```python
from build123d import *

# Parameters (mm, degrees)
SKETCH1_W                                         = 146.05
SKETCH1_H                                         = 95.25
BOSS_EXTRUDE1_DEPTH                               = 3.175
F_6_CLEARANCE_HOLE1_D                             = 4.3053
SKETCH5_R                                         = 6.35
SKETCH5_R_2                                       = 4.7625
CUT_EXTRUDE1_DEPTH                                = 8.4676
CSK_FOR_6_FLAT_HEAD_MACHINE_SCREW_100_D           = 4.3053
CSK_FOR_6_FLAT_HEAD_MACHINE_SCREW_100_CSINK_D     = 7.0866
CSK_FOR_6_FLAT_HEAD_MACHINE_SCREW_100_CSINK_ANGLE = 100
SKETCH8_R                                         = 1.134488875
CUT_EXTRUDE2_DEPTH                                = 4.175


with BuildPart() as part:
    # Sketch1 → Boss-Extrude1 (new body)
    with BuildSketch(Plane.XY):
        with Locations((-73.025, 47.625)):
            Rectangle(SKETCH1_W, SKETCH1_H)
    extrude(amount=-BOSS_EXTRUDE1_DEPTH)

    # #6 Clearance Hole1 (through all)
    with Locations(Plane(origin=(0, 0, -3.175), x_dir=(-1, 0, 0), z_dir=(0, 0, -1))):
        with Locations((4.8895, 80.9625), (141.1605, 80.9625), (141.1605, 14.2875), (4.8895, 14.2875), (46.99, 9.525), (85.725, 9.525), (97.79, 82.55), (46.99, 82.55)):
            Hole(F_6_CLEARANCE_HOLE1_D / 2)

    # Sketch5 → Cut-Extrude1 (cut, through all)
    with BuildSketch(Plane(origin=(0, 0, -7.4676), x_dir=(-1, 0, 0), z_dir=(0, 0, -1))):
        with Locations((30.988, 66.675)):
            Circle(SKETCH5_R)
        with Locations((113.03, 66.675)):
            Circle(SKETCH5_R)
        with Locations((64.5795, 20.955)):
            Circle(SKETCH5_R)
        with Locations((31.242, 20.955)):
            Circle(SKETCH5_R)
        with Locations((73.025, 68.326)):
            Circle(SKETCH5_R_2)
        with Locations((104.775, 21.59)):
            Circle(SKETCH5_R_2)
    extrude(amount=-CUT_EXTRUDE1_DEPTH, mode=Mode.SUBTRACT)

    # CSK for #6 Flat Head Machine Screw (100)1 (through all)
    with Locations(Plane(origin=(0, 0, -3.175), x_dir=(-1, 0, 0), z_dir=(0, 0, -1))):
        with Locations((90.4875, 43.815), (90.4875, 18.415), (119.0625, 7.636172046), (119.0625, 18.415), (119.0625, 43.815), (128.5875, 43.815)):
            CounterSinkHole(CSK_FOR_6_FLAT_HEAD_MACHINE_SCREW_100_D / 2, CSK_FOR_6_FLAT_HEAD_MACHINE_SCREW_100_CSINK_D / 2, counter_sink_angle=CSK_FOR_6_FLAT_HEAD_MACHINE_SCREW_100_CSINK_ANGLE)

    # Sketch8 → Cut-Extrude2 (cut, through all)
    with BuildSketch(Plane.XY):
        with Locations((-70.012401844, 73.606641948)):
            Circle(SKETCH8_R)
    extrude(amount=-CUT_EXTRUDE2_DEPTH, mode=Mode.SUBTRACT)


solid = part.part
```
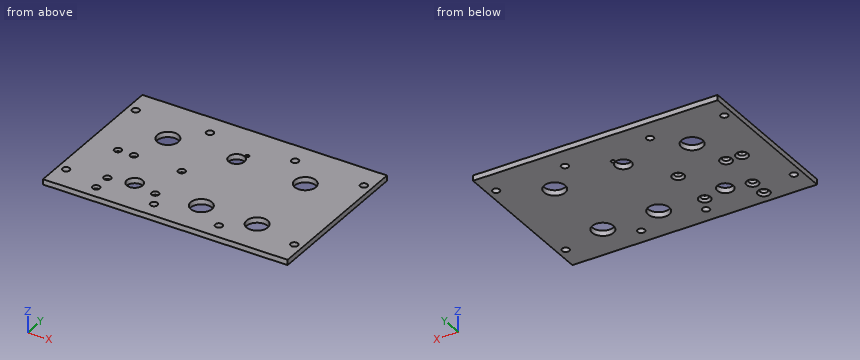
Verification items for the finished model (mm, model axes). Coordinates: 2 decimals unless noted, no trailing zeros. Order: outer loops, then holes, each group sorted by start corner. A loop starts at its lowest first (then second) coordinate and runs counter-clockwise, first axis right, second up. Notation, with made-up numbers: (-38.75, 70.25) -> (6.25, 70.25) arc R21 cw to (6.25, 87.25) -> close; hole circle Ø9 at (-26, 33). An arc over 180 degrees is marked (long way). Put each result on its own line as item: value. Start each with the question number.
1) Cross-section at B-B (y = 24). Enter the section's corners in (x, z) (3 decimals).
2) Cross-section at A-A (x = -97.79). Enter the section's corners in (y, z) (3 decimals), plus the area to 3 significant figures.
3) Material ranges on L1, parallel to X at y = 68, z = -2.05; L2, parallel to Y at x = -25.5, z = -1.7; L3, parallel to X at y = 63, z = -0.4, recorded low to high.
4) Cross-section at D-D (x = -113.03). Enter the section's corners in (y, z) (3 decimals).
5) Go/stop test with a flat-tipped pin: pin 1 (16.5 mm diameter, centred on x = -64.58, y = 20.96, fed in from +Z). Record where the tip stops, or that it passes through.
6) Cross-section at C-C (z = -2.65). State how many separate pieces and enclosed holes the cut face has, plus the area to 3 significant figures.
Geometry check:
1. outline: (-146.05, -3.175) -> (-108.883, -3.175) -> (-108.883, 0) -> (-146.05, 0) -> close; (-100.667, -3.175) -> (-70.152, -3.175) -> (-70.152, 0) -> (-100.667, 0) -> close; (-59.007, -3.175) -> (-36.814, -3.175) -> (-36.814, 0) -> (-59.007, 0) -> close; (-25.67, -3.175) -> (0, -3.175) -> (0, 0) -> (-25.67, 0) -> close
2. outline: (0, -3.175) -> (80.397, -3.175) -> (80.397, 0) -> (0, 0) -> close; (84.703, -3.175) -> (95.25, -3.175) -> (95.25, 0) -> (84.703, 0) -> close
2. area: 289 mm^2
3. L1: x = -146.05 to -119.24, -106.82 to -77.78, -68.27 to -37.2, -24.78 to 0
3. L2: y = 0 to 18.24, 23.67 to 63.48, 69.87 to 95.25
3. L3: x = -146.05 to -118.21, -107.85 to -36.17, -25.81 to 0
4. outline: (0, -3.175) -> (60.325, -3.175) -> (60.325, 0) -> (0, 0) -> close; (73.025, -3.175) -> (95.25, -3.175) -> (95.25, 0) -> (73.025, 0) -> close
5. pin 1: stops at z = 0
6. separate pieces: 1
6. enclosed holes: 21
6. area: 13,000 mm^2
